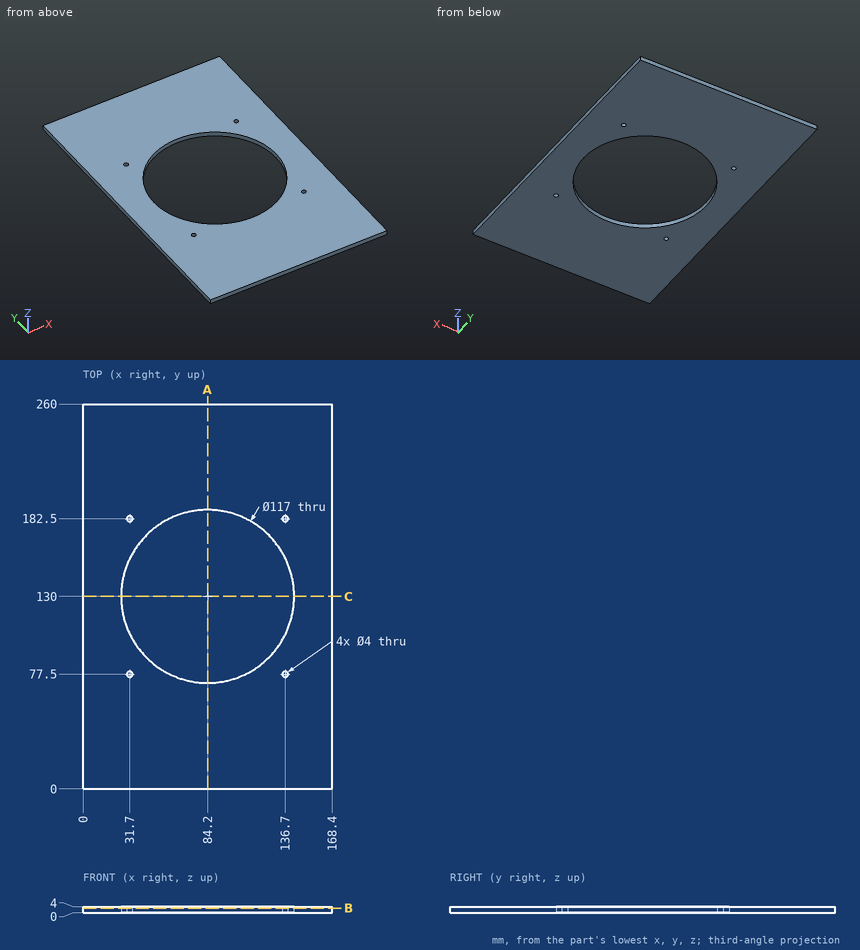
Part print with two shaded views. Sizes in mm from the minimum x, y, z corner. Round coordinates to 2 decimals unless told otherwise and drop trailing zeros. Loops run counter-clockwise (first coordinate to the right, second up) from the corner with the lowest first, then second, coordinate; pieces in that order, holes last. Notation, with made-up numbers: M 36,-8.5 L 56,-8.5 A28 cw 56,24.5 Z; hole C -2.5,52 d7. An arc over 180 degrees is marked long. Return JSON: item names as keys, results as strings. Group by question number.
(1) Drop a flat-ended pin along its axis: P1, Ø12, axis at x = 126, y = 98.5, coming from the +Z side. Give the stop position or say it passes through.
(2) Saw through at B-B, the plane z = 3.05. List the corners of the cut face in (x, y).
(3) Wall check: probe 1 along Y at (x, z) = (63, 3.2); probe 2 along X at (y, z) = (77.5, 2.95); probe 3 along Y at (x, z) = (136.7, 1.35). Give the ranges that are in metal, low to high. Write a range as [from, to].
(4) Saw through at C-C, the plane y = 130. List the corners of the cut face in (x, z).
(5) Saw through at A-A, the plane x = 84.2. List the corners of the cut face in (y, z), and give its area (3 significant figures).
Answer list:
{
 "1": {"P1": "through"},
 "2": {"outline": "M 0,0 L 168.4,0 L 168.4,260 L 0,260 Z; hole C 84.2,130 d117; hole C 31.7,77.5 d4; hole C 31.7,182.5 d4; hole C 136.7,77.5 d4; hole C 136.7,182.5 d4"},
 "3": {"probe 1": "[0, 75.48], [184.52, 260]", "probe 2": "[0, 29.7], [33.7, 58.39], [110.01, 134.7], [138.7, 168.4]", "probe 3": "[0, 75.5], [79.5, 104.19], [155.81, 180.5], [184.5, 260]"},
 "4": {"outline": "M 0,0 L 25.7,0 L 25.7,4 L 0,4 Z; M 142.7,0 L 168.4,0 L 168.4,4 L 142.7,4 Z"},
 "5": {"outline": "M 0,0 L 71.5,0 L 71.5,4 L 0,4 Z; M 188.5,0 L 260,0 L 260,4 L 188.5,4 Z", "area": "572 mm2"}
}
